from build123d import *

# Parameters (mm, degrees)
SKETCH1_R           = 30
SKETCH1_R_2         = 20
BOSS_EXTRUDE1_DEPTH = 20
BOSS_EXTRUDE2_DEPTH = 2.5


with BuildPart() as part:
    # Sketch1 → Boss-Extrude1 (new, symmetric)
    with BuildSketch(Plane(origin=(0, 0, 0), x_dir=(1, 0, 0), z_dir=(0, 1, 0))):
        with Locations(Location((0, 0, 0), (0, 0, 270))):
            Circle(SKETCH1_R)
        with Locations(Location((0, 0, 0), (0, 0, 270))):
            Circle(SKETCH1_R_2, mode=Mode.SUBTRACT)
    extrude(amount=BOSS_EXTRUDE1_DEPTH, both=True)

    # Sketch2 → Boss-Extrude2 (add, symmetric)
    with BuildSketch(Plane(origin=(0, 0, 0), x_dir=(1, 0, 0), z_dir=(0, 1, 0))):
        with BuildLine():
            Line((28.120382297, 10.451990215), (55.080308758, 10.451990215))
            Line((55.080308758, 10.451990215), (55.080308758, 5.574382734))
            Line((55.080308758, 5.574382734), (71.919231742, 5.574382734))
            Line((71.919231742, 5.574382734), (71.919231742, 36.006171261))
            Line((71.919231742, 36.006171261), (80.002186763, 45.140832286))
            Line((80.002186763, 45.140832286), (101.742384499, 45.140832286))
            Line((101.742384499, 45.140832286), (101.742384499, -45.140832286))
            Line((101.742384499, -45.140832286), (80.002186763, -45.140832286))
            Line((80.002186763, -45.140832286), (71.919231742, -36.006171261))
            Line((71.919231742, -36.006171261), (71.919231742, -5.574382734))
            Line((71.919231742, -5.574382734), (55.080308758, -5.574382734))
            Line((55.080308758, -5.574382734), (55.080308758, -10.451990215))
            Line((55.080308758, -10.451990215), (28.120382297, -10.451990215))
            ThreePointArc((28.120382297, -10.451990215), (30, 0), (28.120382297, 10.451990215))
        make_face()
    extrude(amount=BOSS_EXTRUDE2_DEPTH, both=True)


solid = part.part
Check sheet for the modelled part. Datum: model origin and axes. Units: mm. A direction names the side the tool comes from. Round coordinates to 2 decimals unless told otherwise and drop trailing zeros. Order: outer loops, then holes, each group sorted by start corner. A loop starts at its lowest first (then second) coordinate and runs counter-clockwise, first axis right, second up.
Q1. Cross-section at D-D, the plane y = 4.5. Enter the section's corners in (x, z), plus the area to 3 significant figures.
Filled sheet:
outline: circle Ø60 at (0, 0); hole circle Ø40 at (0, 0)
area: 1,570 mm2
Q2. Draft check along Z on faces 4 (the face through (41, 0, -10.452)), 5 (the face through (55.08, 0, -8)), 6 (the face through (64, 0, 5.574)), 7 (the face through (-19.524, -0.28, -4.336)). Enter one of: pulls with the +Z half, pulls with the -Z half, needs draft (parallel to the pull), parting line crosses it, or undercut.
Filled sheet:
face 4: pulls with the -Z half
face 5: needs draft
face 6: pulls with the +Z half
face 7: undercut
Q3. Set-up check for faces 1 (the face through (55.08, 0, 8)), 2 (the face through (75.904, 0.035, -40.51)), 3 (the face through (71.919, 0, -21)): record each of +Z, -Z, +X, -X, +Y, -Y from which the full face is reachable in a straight line by a thin tool's end or side.
Filled sheet:
face 1: +Z, +Y, -Y
face 2: -Z, -X, +Y, -Y
face 3: -Z, +Y, -Y
Q4. Depth check by flat-ended pin: P1, Ø4, axis at x = 42, y = -1, coming from the +Z side; P2, Ø6, axis at x = 78.5, y = -3.5, coming from the +Z side; P3, Ø2.5, axis at x = 62, y = -0.5, coming from the -Z side; P4, Ø4, axis at x = 21, y = -5.5, coming from the +Z side. Enter the tip coordinate at first touch or a pass-through.
Filled sheet:
P1: stops at z = 10.45
P2: stops at z = 45.14
P3: stops at z = -5.57
P4: stops at z = 23.22
Q5. Cross-section at B-B, the plane z = 0. Enter the section's corners in (x, y).
Filled sheet:
outline: (-30, -20) - (-20, -20) - (-20, 20) - (-30, 20) - close; (20, -20) - (30, -20) - (30, -2.5) - (101.74, -2.5) - (101.74, 2.5) - (30, 2.5) - (30, 20) - (20, 20) - close
Q6. Cross-section at A-A, the plane x = 0. Enter the section's corners in (y, z), plus the area to 3 significant figures.
Filled sheet:
outline: (-20, -30) - (20, -30) - (20, -20) - (-20, -20) - close; (-20, 20) - (20, 20) - (20, 30) - (-20, 30) - close
area: 800 mm2
Q7. Scan lines: L1, parallel to X at y = 1, z = 0; L2, parallel to Y at x = 79, z = 15; L3, parallel to X at y = 3, z = -18. Record each from-to range of solid material in increasing order.
Filled sheet:
L1: x = -30 to -20, 20 to 101.74
L2: y = -2.5 to 2.5
L3: x = -24 to -8.72, 8.72 to 24
Q8. Cross-section at C-C, the plane z = 14. Enter the section's corners in (x, y), plus the area to 3 significant figures.
Filled sheet:
outline: (-26.53, -20) - (-14.28, -20) - (-14.28, 20) - (-26.53, 20) - close; (14.28, -20) - (26.53, -20) - (26.53, 20) - (14.28, 20) - close; (71.92, -2.5) - (101.74, -2.5) - (101.74, 2.5) - (71.92, 2.5) - close
area: 1,130 mm2
